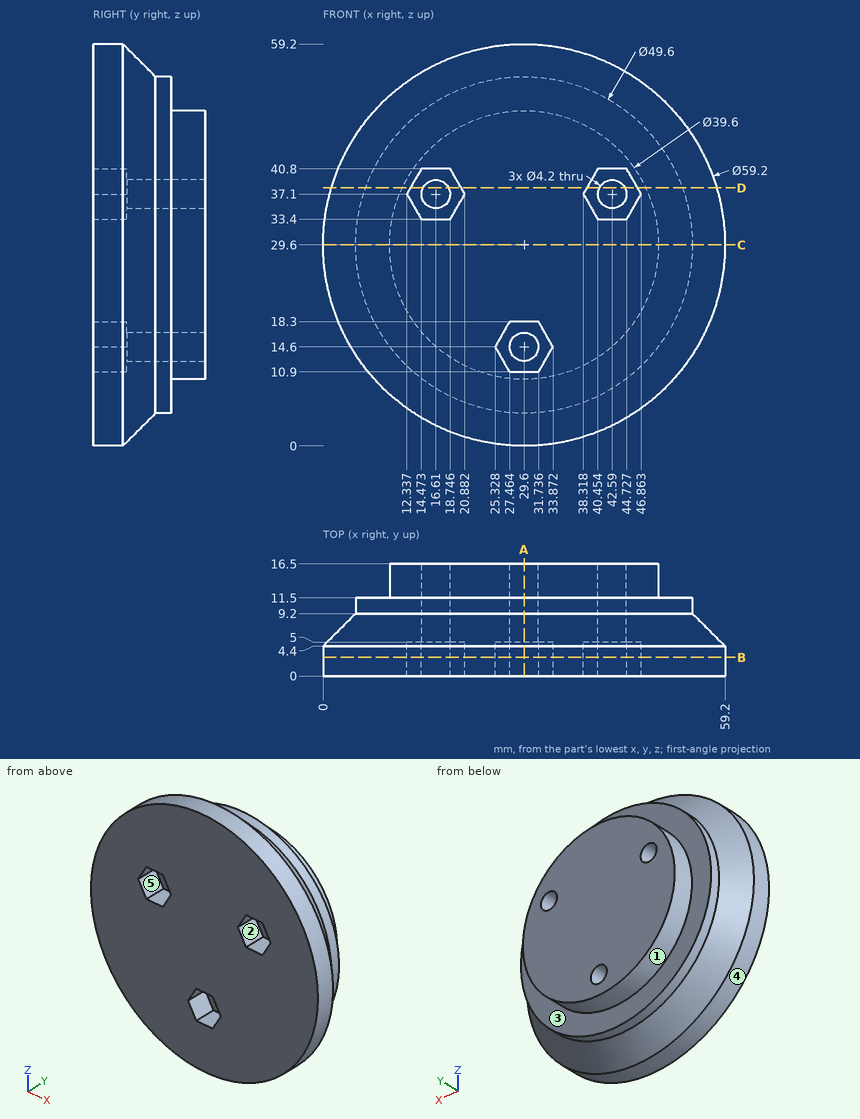
Input: dimensioned drawing with shaded views. Units: mm. Origin: part minimum x, y, z. A direction names the side the tool comes from. Round coordinates to 2 decimals unless told otherwise and drop trailing zeros. Loops run counter-clockwise (first coordinate to the right, second up) from the corner with the lowest first, then second, coordinate; pieces in that order, holes last. Notation, with made-up numbers: M 66,54.5 L 70,54.5 A16 ccw 70,66.5 Z; hole C 14,51.25 d5. An arc over 180 degrees is marked long. Return JSON: item names as keys, results as strings. Group by question number.
1. Reachability of the marked faces 4 and 5 from +Z, -Z, +X, -X, +Y, -Y: full face, straight path, thin tool, end or side. Return the list, or none.
2. Section query B-B on y = 2.75. Output: boundary loops of the cut face in (x, z) (1 decimal).
3. Section query C-C on z = 29.6. Output: boundary loops of the cut face in (x, y), and give its area (3 significant figures).
4. Section query D-D on z = 38. State how many separate pieces and enclosed holes the cut face has.
5. Pin query (flat end, axial travel): pin 1 (10 mm diameter, centred on x = 25.5, z = 12.5, fed in from -Y); pin 2 (4 mm diameter, centred on x = 48.5, y = 8.5, fed in from +Z); pin 3 (4 mm diameter, centred on y = 12.5, z = 33, fed in from -X); pin 4 (1.5 mm diameter, centred on x = 24, y = 4, fed in from -Z). Return the tip coordinate at first contact, or that it passes through.
6. Material intervals for line 1 along X through (y, z) = (8.25, 36); line 2 along Z through (x, y) = (30.5, 2.75); line 3 along X through (y, z) = (12.5, 37.1) (1 decimal), sorted ascending. Write a range as from..to.
7. Section query A-A on x = 29.6. Output: boundary loops of the cut face in (y, z).
8. Mould query, pull axis X, two halves, no side actions, for the marked faces 1, 2 and 3. Classes: released by +X, released by -X, zero draft, split by the parting line, or undercut.
Checks:
{
 "1": {"face 4": "+Y, -Y", "face 5": "-Y"},
 "2": {"outline": "C 29.6,29.6 d59.2; hole M 12.3,37.1 L 14.5,33.4 L 18.7,33.4 L 20.9,37.1 L 18.7,40.8 L 14.5,40.8 Z; hole M 25.3,14.6 L 27.5,10.9 L 31.7,10.9 L 33.9,14.6 L 31.7,18.3 L 27.5,18.3 Z; hole M 38.3,37.1 L 40.5,33.4 L 44.7,33.4 L 46.9,37.1 L 44.7,40.8 L 40.5,40.8 Z"},
 "3": {"outline": "M 0,0 L 59.2,0 L 59.2,4.4 L 54.4,9.2 L 54.4,11.5 L 49.4,11.5 L 49.4,16.5 L 9.8,16.5 L 9.8,11.5 L 4.8,11.5 L 4.8,9.2 L 0,4.4 Z", "area": "834 mm²"},
 "4": {"separate pieces": "3", "enclosed holes": "0"},
 "5": {"pin 1": "stops at y = 0", "pin 2": "stops at z = 50.13", "pin 3": "stops at x = 4.86", "pin 4": "stops at z = 0.4"},
 "6": {"line 1": "x = 4.66..14.82, 18.4..40.8, 44.38..54.54", "line 2": "z = 0.01..10.9, 18.3..59.19", "line 3": "x = 11.3..14.5, 18.7..40.5, 44.7..47.9"},
 "7": {"outline": "M 0,0 L 4.4,0 L 9.2,4.8 L 11.5,4.8 L 11.5,9.8 L 16.5,9.8 L 16.5,12.5 L 5,12.5 L 5,10.9 L 0,10.9 Z; M 0,18.3 L 5,18.3 L 5,16.7 L 16.5,16.7 L 16.5,49.4 L 11.5,49.4 L 11.5,54.4 L 9.2,54.4 L 4.4,59.2 L 0,59.2 Z"},
 "8": {"face 1": "split by the parting line", "face 2": "undercut", "face 3": "zero draft"}
}
